from build123d import *

# Parameters (mm, degrees)
SKETCH_1_W      = 4.4
SKETCH_1_H      = 20.4
SKETCH_1_W_2    = 30.4
SKETCH_1_H_2    = 4.4
EXTRUDE_1_DEPTH = 4


with BuildPart() as part:
    # Эскиз1 → Бобышка-Вытянуть1 (new body)
    with BuildSketch(Plane.XY):
        Polygon((0, 0), (0, 150), (200, 100), (200, 0), align=None)
        with Locations((189, 29.8)):
            Rectangle(SKETCH_1_W, SKETCH_1_H, mode=Mode.SUBTRACT)
        with Locations((155, 8)):
            Rectangle(SKETCH_1_W_2, SKETCH_1_H_2, mode=Mode.SUBTRACT)
        with Locations((45, 8)):
            Rectangle(SKETCH_1_W_2, SKETCH_1_H_2, mode=Mode.SUBTRACT)
        with Locations((8, 109.8)):
            Rectangle(SKETCH_1_W, SKETCH_1_H, mode=Mode.SUBTRACT)
        with Locations((189, 80.8)):
            Rectangle(SKETCH_1_W, SKETCH_1_H, mode=Mode.SUBTRACT)
        with Locations((8, 29.8)):
            Rectangle(SKETCH_1_W, SKETCH_1_H, mode=Mode.SUBTRACT)
    extrude(amount=EXTRUDE_1_DEPTH)


solid = part.part
The listing builds one solid part. Answer for the finished solid, in the listing's coordinates (mm). Coordinates: 2 decimals unless noted, no trailing zeros. Write each loop counter-clockwise with the first axis right and the second up, starting at its lowest first coordinate (ties: lowest second). Pieces come first, ordered by that corner, then holes. Notation, with made-up numbers: (64.5, 8.5) -> (87.5, 8.5) arc R30 ccw to (87.5, 31.5) -> close; hole circle Ø1 at (-6.5, 15). An arc over 180 degrees is marked (long way). One line per question, with ' | ' between items.
1. Section D-D (x = 142.5) is taken. Determine the outline of the cut face in (y, z) (3 decimals), and give its area (3 significant figures).
Verdict:
outline: (0, 0) -> (5.8, 0) -> (5.8, 4) -> (0, 4) -> close; (10.2, 0) -> (114.375, 0) -> (114.375, 4) -> (10.2, 4) -> close | area: 440 mm^2
2. Given pin 1 Ø2 at (x, z) = (156.5, 2.5) entering from +Y (3 decimals); pin 2 Ø1.2 at (x, z) = (7.5, 2) entering from +Y (3 decimals), each flat-ended and moving along its own axis, determine where each tip first touches the part or whether it passes through.
Verdict:
pin 1: stops at y = 111.125 | pin 2: stops at y = 148.275
3. Straight lines are drawn through the part: line 1 (X direction, y = 38, z = 1.3); line 2 (X direction, y = 85, z = 1.5); line 3 (X direction, y = 7.5, z = 1.3). For each, find the intervals that lie inside material, in ascending order.
Verdict:
line 1: x = 0 to 5.8, 10.2 to 186.8, 191.2 to 200 | line 2: x = 0 to 186.8, 191.2 to 200 | line 3: x = 0 to 29.8, 60.2 to 139.8, 170.2 to 200
4. Section C-C (y = 23) is taken. Determine the outline of the cut face in (x, z), and give its area (3 significant figures).
Verdict:
outline: (0, 0) -> (5.8, 0) -> (5.8, 4) -> (0, 4) -> close; (10.2, 0) -> (186.8, 0) -> (186.8, 4) -> (10.2, 4) -> close; (191.2, 0) -> (200, 0) -> (200, 4) -> (191.2, 4) -> close | area: 765 mm^2
5. Section B-B (z = 2.1) is taken. Determine the outline of the cut face in (x, y).
Verdict:
outline: (0, 0) -> (200, 0) -> (200, 100) -> (0, 150) -> close; hole (5.8, 19.6) -> (10.2, 19.6) -> (10.2, 40) -> (5.8, 40) -> close; hole (5.8, 99.6) -> (10.2, 99.6) -> (10.2, 120) -> (5.8, 120) -> close; hole (29.8, 5.8) -> (60.2, 5.8) -> (60.2, 10.2) -> (29.8, 10.2) -> close; hole (139.8, 5.8) -> (170.2, 5.8) -> (170.2, 10.2) -> (139.8, 10.2) -> close; hole (186.8, 19.6) -> (191.2, 19.6) -> (191.2, 40) -> (186.8, 40) -> close; hole (186.8, 70.6) -> (191.2, 70.6) -> (191.2, 91) -> (186.8, 91) -> close
6. For a pull along Y with two mould halves and no side action, classify faces 1 (the flat face through (5.8, 30, 2)), 2 (the flat face through (101, 59, 4)) as released by +Y, released by -Y, zero draft, split by the parting line, or undercut.
Verdict:
face 1: undercut | face 2: zero draft
7. Section A-A (y = 75.5) is taken. Determine the outline of the cut face in (x, z), and give its area (3 significant figures).
Verdict:
outline: (0, 0) -> (186.8, 0) -> (186.8, 4) -> (0, 4) -> close; (191.2, 0) -> (200, 0) -> (200, 4) -> (191.2, 4) -> close | area: 782 mm^2
